Part model, mm, in its own coordinate system. Face numbers are marked on the shaded views. A direction names the side the tool comes from. Round coordinates to 2 decimals unless told otherwise and drop trailing zeros. Order: outer loops, then holes, each group sorted by start corner. A loop starts at its lowest first (then second) coordinate and runs counter-clockwise, first axis right, second up. Notation, with made-up numbers: (70.25, -33) -> (124.25, -33) arc R23 cw to (124.25, -23) -> close; hole circle Ø3 at (11, 55.5). An arc over 180 degrees is marked (long way). Return JSON: item names as keys, results as strings. Group by question number.
from build123d import *

# Parameters (mm, degrees)
SKETCH_1_R          = 9
EXTRUDE_1_DEPTH     = 8
SKETCH_2_R          = 9
EXTRUDE_2_DEPTH     = 2
SKETCH_3_R          = 6.78
EXTRUDE_3_DEPTH     = 11
SKETCH_4_R          = 9
EXTRUDE_4_DEPTH     = 2
SKETCH_5_R          = 2.5
CUT_EXTRUDE_1_DEPTH = 31


with BuildPart() as part:
    # 草图1 → 凸台-拉伸1 (new body)
    with BuildSketch(Plane(origin=(0, 0, 0), x_dir=(1, 0, 0), z_dir=(0, 1, 0))):
        with Locations(Location((0, 0, 0), (0, 0, 270))):
            Circle(SKETCH_1_R)
    extrude(amount=EXTRUDE_1_DEPTH)

    # 草图2 → 凸台-拉伸2 (add)
    with BuildSketch(Plane(origin=(0, 8, 0), x_dir=(1, 0, 0), z_dir=(0, 1, 0))):
        with Locations(Location((0, 0, 0), (0, 0, 270))):
            Circle(SKETCH_2_R)
    extrude(amount=EXTRUDE_2_DEPTH)

    # 草图3 → 凸台-拉伸3 (add)
    with BuildSketch(Plane(origin=(0, 10, 0), x_dir=(1, 0, 0), z_dir=(0, 1, 0))):
        with Locations(Location((0, 0, 0), (0, 0, 270))):
            Circle(SKETCH_3_R)
    extrude(amount=EXTRUDE_3_DEPTH)

    # 草图4 → 凸台-拉伸4 (add)
    with BuildSketch(Plane(origin=(0, 21, 0), x_dir=(1, 0, 0), z_dir=(0, 1, 0))):
        with Locations(Location((0, 0, 0), (0, 0, 270))):
            Circle(SKETCH_4_R)
    extrude(amount=EXTRUDE_4_DEPTH)

    # 草图5 → 切除-拉伸1 (cut)
    with BuildSketch(Plane(origin=(0, 23, 0), x_dir=(1, 0, 0), z_dir=(0, 1, 0))):
        with Locations(Location((0, 0, 0), (0, 0, 270))):
            Circle(SKETCH_5_R)
    extrude(amount=-CUT_EXTRUDE_1_DEPTH, mode=Mode.SUBTRACT)


solid = part.part
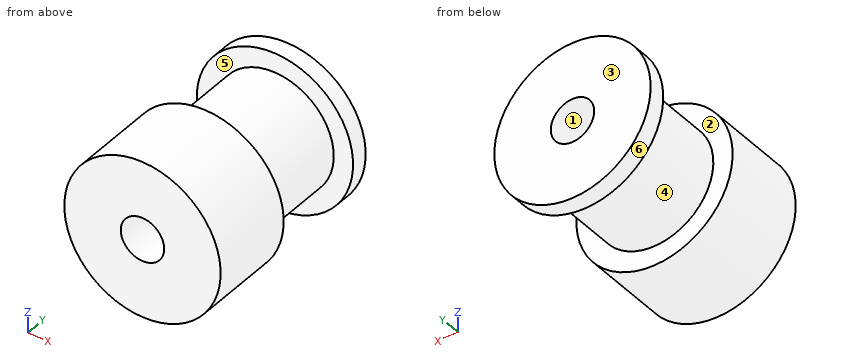
(1) Saw through at B-B, the plane z = -0.25. List the corners of the cut face in (x, y), and give its area (3 significant figures).
(2) Saw through at A-A, the plane x = 0. List the corners of the cut face in (y, z), and give its area (3 significant figures).
(3) Saw through at D-D, the plane z = 3.25. List the corners of the cut face in (x, y).
(4) Tool access for the marked faces 5 and 6: list every direction of +Z, -Z, +X, -X, +Y, -Y with a clear straight run to the whole face (end or side of a thin tool).
(5) Saw through at C-C, the plane x = 4.75. List the corners of the cut face in (y, z), and give its area (3 significant figures).
(6) Probe L1, parallel to Y at x = 1, z = 7; L2, parallel to X at y = 5.5, z = 0; L3, parallel to X at y = 11.25, z = 0. List the from-to ranges inside material, lowest first. Write a range as [from, to].
(7) Mould opens along Y. For the marked faces 1, 2, 3 and 4 say: pulls with the +Y half, pulls with the -Y half, needs draft (parallel to the pull), parting line crosses it, or undercut.
(8) Pin check, flat tips, straight feed: P1, Ø4, axis at x = 7, y = 8, coming from the -Z side; P2, Ø10, axis at y = 12.5, z = -6.5, coming from the +X side; P3, Ø5, axis at y = 8, z = 5, coming from the -X side; P4, Ø5, axis at x = 1.5, z = 2.5, coming from the -Y side. Stop position of each tip, or through.
Results are:
{
 "1": {"outline": "(-9, 0) -> (-2.49, 0) -> (-2.49, 23) -> (-9, 23) -> (-9, 21) -> (-6.78, 21) -> (-6.78, 10) -> (-9, 10) -> close; (2.49, 0) -> (9, 0) -> (9, 10) -> (6.78, 10) -> (6.78, 21) -> (9, 21) -> (9, 23) -> (2.49, 23) -> close", "area": "251 mm^2"},
 "2": {"outline": "(0, -9) -> (10, -9) -> (10, -6.78) -> (21, -6.78) -> (21, -9) -> (23, -9) -> (23, -2.5) -> (0, -2.5) -> close; (0, 2.5) -> (23, 2.5) -> (23, 9) -> (21, 9) -> (21, 6.78) -> (10, 6.78) -> (10, 9) -> (0, 9) -> close", "area": "250 mm^2"},
 "3": {"outline": "(-8.39, 0) -> (8.39, 0) -> (8.39, 10) -> (5.95, 10) -> (5.95, 21) -> (8.39, 21) -> (8.39, 23) -> (-8.39, 23) -> (-8.39, 21) -> (-5.95, 21) -> (-5.95, 10) -> (-8.39, 10) -> close"},
 "4": {"face 5": "none", "face 6": "+Y, -Y"},
 "5": {"outline": "(0, -7.64) -> (10, -7.64) -> (10, -4.84) -> (21, -4.84) -> (21, -7.64) -> (23, -7.64) -> (23, 7.64) -> (21, 7.64) -> (21, 4.84) -> (10, 4.84) -> (10, 7.64) -> (0, 7.64) -> close", "area": "290 mm^2"},
 "6": {"L1": "y = [0, 10], [21, 23]", "L2": "x = [-9, -2.5], [2.5, 9]", "L3": "x = [-6.78, -2.5], [2.5, 6.78]"},
 "7": {"face 1": "needs draft", "face 2": "undercut", "face 3": "pulls with the +Y half", "face 4": "undercut"},
 "8": {"P1": "stops at z = -7.48", "P2": "stops at x = 8.73", "P3": "stops at x = -8.65", "P4": "stops at y = 0"}
}
